from build123d import *

# Parameters (mm, degrees)
BOSS_EXTRUDE1_DEPTH   = 5
CUT_EXTRUDE1_REACH    = 123.758
SKETCH2_R             = 1.5
SKETCH2_R_2           = 1
BODY_MOVE_COPY1_ANGLE = 90
SKETCH19_R            = 2.25
SKETCH19_W            = 40.05
SKETCH19_H            = 21
CUT_EXTRUDE9_DEPTH    = 122.757956619


with BuildPart() as part:
    # Sketch1 → Boss-Extrude1 (new body)
    with BuildSketch(Plane(origin=(0, 0, 0), x_dir=(1, 0, 0), z_dir=(0, 1, 0))):
        with BuildLine():
            Line((100, -20), (0, -20))
            ThreePointArc((0, -20), (-20, 0), (0, 20))
            Line((0, 20), (100, 20))
            ThreePointArc((100, 20), (120, 0), (100, -20))
        make_face()
    extrude(amount=BOSS_EXTRUDE1_DEPTH)

    # Sketch2 → Cut-Extrude1 (cut, up to next)
    with BuildSketch(Plane(origin=(0, 5, 0), x_dir=(1, 0, 0), z_dir=(0, 1, 0)), mode=Mode.PRIVATE) as cut_extrude1_sk1:
        with Locations(Location((0, 0, 0), (0, 0, 270))):
            Circle(SKETCH2_R)
    cut_extrude1_tool1 = extrude(cut_extrude1_sk1.sketch, amount=-CUT_EXTRUDE1_REACH, mode=Mode.PRIVATE) & part.part
    # Sketch2 → Cut-Extrude1 (cut, up to next)
    with BuildSketch(Plane(origin=(0, 5, 0), x_dir=(1, 0, 0), z_dir=(0, 1, 0)), mode=Mode.PRIVATE) as cut_extrude1_sk2:
        with Locations(Location((0, 7, 0), (0, 0, 270))):
            Circle(SKETCH2_R_2)
    cut_extrude1_tool2 = extrude(cut_extrude1_sk2.sketch, amount=-CUT_EXTRUDE1_REACH, mode=Mode.PRIVATE) & part.part
    # Sketch2 → Cut-Extrude1 (cut, up to next)
    with BuildSketch(Plane(origin=(0, 5, 0), x_dir=(1, 0, 0), z_dir=(0, 1, 0)), mode=Mode.PRIVATE) as cut_extrude1_sk3:
        with Locations(Location((7.001, 0.001, 0), (0, 0, 270))):
            Circle(SKETCH2_R_2)
    cut_extrude1_tool3 = extrude(cut_extrude1_sk3.sketch, amount=-CUT_EXTRUDE1_REACH, mode=Mode.PRIVATE) & part.part
    # Sketch2 → Cut-Extrude1 (cut, up to next)
    with BuildSketch(Plane(origin=(0, 5, 0), x_dir=(1, 0, 0), z_dir=(0, 1, 0)), mode=Mode.PRIVATE) as cut_extrude1_sk4:
        with Locations(Location((0.002, -7, 0), (0, 0, 270))):
            Circle(SKETCH2_R_2)
    cut_extrude1_tool4 = extrude(cut_extrude1_sk4.sketch, amount=-CUT_EXTRUDE1_REACH, mode=Mode.PRIVATE) & part.part
    # Sketch2 → Cut-Extrude1 (cut, up to next)
    with BuildSketch(Plane(origin=(0, 5, 0), x_dir=(1, 0, 0), z_dir=(0, 1, 0)), mode=Mode.PRIVATE) as cut_extrude1_sk5:
        with Locations(Location((-6.999, -0.001, 0), (0, 0, 270))):
            Circle(SKETCH2_R_2)
    cut_extrude1_tool5 = extrude(cut_extrude1_sk5.sketch, amount=-CUT_EXTRUDE1_REACH, mode=Mode.PRIVATE) & part.part
    add(cut_extrude1_tool1.solids().sort_by_distance((0, 5, 0))[0], mode=Mode.SUBTRACT)
    add(cut_extrude1_tool2.solids().sort_by_distance((0, 5, -7))[0], mode=Mode.SUBTRACT)
    add(cut_extrude1_tool3.solids().sort_by_distance((7.001, 5, -0.001))[0], mode=Mode.SUBTRACT)
    add(cut_extrude1_tool4.solids().sort_by_distance((0.002, 5, 7))[0], mode=Mode.SUBTRACT)
    add(cut_extrude1_tool5.solids().sort_by_distance((-6.999, 5, 0.001))[0], mode=Mode.SUBTRACT)


with BuildPart() as part_1:
    # Body-Move/Copy1: moved
    add(part.part.rotate(Axis((0, 0, 0), (1, 0, 0)), BODY_MOVE_COPY1_ANGLE))

    # Sketch19 → Cut-Extrude9 (cut, through all)
    with BuildSketch(Plane.XY.offset(5)):
        with Locations((114.4, -5)):
            Circle(SKETCH19_R)
        with Locations(Location((114.4, 5, 0), (0, 0, 180))):
            Circle(SKETCH19_R)
        with Locations(Location((65.6, 5, 0), (0, 0, 180))):
            Circle(SKETCH19_R)
        with Locations((65.6, -5)):
            Circle(SKETCH19_R)
        with Locations((90, 0)):
            Rectangle(SKETCH19_W, SKETCH19_H)
    extrude(amount=-CUT_EXTRUDE9_DEPTH, mode=Mode.SUBTRACT)


with BuildPart() as part_2:
    # Body-Move/Copy2: moved
    add(part_1.part.moved(Location((0, 0, -5))))


solid = part_2.part
Could you check a few things on this model? Use its own coordinates, in mm. A direction names the side the tool comes from. Coordinates: 2 decimals unless noted, no trailing zeros. Order: outer loops, then holes, each group sorted by start corner. A loop starts at its lowest first (then second) coordinate and runs counter-clockwise, first axis right, second up. Notation, with made-up numbers: (72.25, 47) - (120.25, 47) arc R29 cw to (120.25, 67) - close; hole circle Ø9 at (15, -4). An arc over 180 degrees is marked (long way). Answer in a Markdown table with one row per item. Add a question column.
(1) If we section it at B-B, the plane z = -2.65: State how many separate pieces and enclosed holes the cut face has, then the cut area to 3 significant figures.
(2) If we section it at A-A, the plane x = 65.6: Please give me the cut outline in (y, z), then the cut area to 3 significant figures.
(3) On a 3-axis mill with a long thin cutter (end or side, diameter ignored), from which of +Z, -Z, +X, -X, +Y, -Y can I reach the whole of each face in a straight line? I mean faces 1 (the face through (69.975, 0, -2)), 2 (the face through (49, 20, -3)). Say none if no direction works.
(4) If we section it at C-C, the plane x = -10: Please give me the cut outline in (y, z), then the cut area to 3 significant figures.
(5) If we mould it in two halves opening along Y, with no side actions, what happens to faces 3 (the face through (110.025, 0, -2)), 4 (the face through (35, 0, -5)), 5 (the face through (120, 0, -3))? For each: released by +Y, released by -Y, zero draft, split by the parting line, or undercut.
(6) Will these pins go through, and if not, where does the flat tip stop? pin 1 (6 mm diameter, centred on x = 65.6, y = -5, fed in from +Z); pin 2 (1.2 mm diameter, centred on x = 0.002, y = -7, fed in from +Z); pin 3 (1.5 mm diameter, centred on y = 4, z = -2.5, fed in from -X); pin 4 (1.5 mm diameter, centred on y = 5, z = -3.5, fed in from +X).
(7) I need wall thicknesses on L1, parallel to Y at x = 65.6, z = -2.65; L2, parallel to X at y = 0, z = -1.75 (3 decimals); L3, parallel to Y at x = 92.5, z = -2.2. Which ranges of each line are inside material? Lowest first, please.
Results are:
| question | item | result |
|---|---|---|
| 1 | separate pieces | 1 |
| 1 | enclosed holes | 10 |
| 1 | area | 4,330 mm2 |
| 2 | outline | (-20, -5) - (-7.25, -5) - (-7.25, 0) - (-20, 0) - close; (-2.75, -5) - (2.75, -5) - (2.75, 0) - (-2.75, 0) - close; (7.25, -5) - (20, -5) - (20, 0) - (7.25, 0) - close |
| 2 | area | 155 mm2 |
| 3 | face 1 | +Z, -Z |
| 3 | face 2 | +Z, -Z, +X, -X, +Y |
| 4 | outline | (-17.32, -5) - (17.32, -5) - (17.32, 0) - (-17.32, 0) - close |
| 4 | area | 173 mm2 |
| 5 | face 3 | undercut |
| 5 | face 4 | zero draft |
| 5 | face 5 | split by the parting line |
| 6 | pin 1 | stops at z = 0 |
| 6 | pin 2 | passes through |
| 6 | pin 3 | stops at x = -19.73 |
| 6 | pin 4 | stops at x = 119.54 |
| 7 | L1 | y = -20 to -7.25, -2.75 to 2.75, 7.25 to 20 |
| 7 | L2 | x = -20 to -7.999, -5.999 to -1.5, 1.5 to 6.001, 8.001 to 69.975, 110.025 to 120 |
| 7 | L3 | y = -20 to -10.5, 10.5 to 20 |
